Geometry: final body of the model. Coordinates: model frame, mm. Face numbers are marked on the shaded views. Give positions to 0.01 mm unless a question says otherwise; leave off trailing zeros. Order: outer loops, then holes, each group sorted by start corner. A loop starts at its lowest first (then second) coordinate and runs counter-clockwise, first axis right, second up. Notation, with made-up numbers: M 6.5,28 L 30.5,28 A29 cw 30.5,48 Z; hole C -3.5,34 d5. An arc over 180 degrees is marked long. Use CSV: the item, a comma, the result in double quotes.
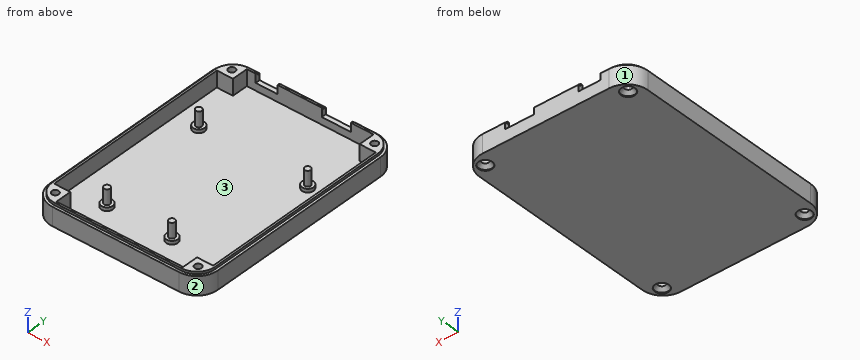
```python
from build123d import *

# Parameters (mm, degrees)
F1_DEPTH  = 2
F2_R      = 2.5
F3_DEPTH  = 1.5
F4_R      = 1.3
F5_DEPTH  = 1.5
F7_DEPTH  = 7
F8_R      = 1.5
F9_DEPTH  = 10
F10_W     = 12.6
F10_H     = 2
F10_W_2   = 9.5
F11_DEPTH = 3.8
F12_R     = 3
F13_DEPTH = 0.4
F14_SIZE  = 1.49999
F15_W     = 19.2
F15_H     = 1.1
F16_DEPTH = 1
F17_DEPTH = 5


# Not quite as in the source:
# - a fillet or chamfer is up to 0.001 mm smaller than in the source, because OpenCascade refuses the exact size


with BuildPart() as f1:
    # F0 (on Top) → F1 (new body)
    with BuildSketch(Plane.XY):
        with BuildLine():
            Line((27.5, 63.5), (-27.5, 63.5))
            ThreePointArc((-27.5, 63.5), (-33.8639610307, 60.8639610307), (-36.5, 54.5))
            Line((-36.5, 54.5), (-36.5, -27.5))
            ThreePointArc((-36.5, -27.5), (-33.8639610307, -33.8639610307), (-27.5, -36.5))
            Line((-27.5, -36.5), (27.5, -36.5))
            ThreePointArc((27.5, -36.5), (33.8639610307, -33.8639610307), (36.5, -27.5))
            Line((36.5, -27.5), (36.5, 54.5))
            ThreePointArc((36.5, 54.5), (33.8639610307, 60.8639610307), (27.5, 63.5))
        make_face()
    extrude(amount=F1_DEPTH)

    # F2 (on face) → F3 (join)
    with BuildSketch(Plane.XY.offset(2)):
        with Locations((-19.24, -18.6)):
            Circle(F2_R)
        with Locations((8.96, -18.6)):
            Circle(F2_R)
        with Locations((24.16, 32.2)):
            Circle(F2_R)
        with Locations((-24.24, 33.5)):
            Circle(F2_R)
    extrude(amount=F3_DEPTH)

    # F4 (on face) → F5 (join)
    with BuildSketch(Plane.XY.offset(3.5)):
        with Locations((-19.24, -18.6)):
            Circle(F4_R)
        with Locations((8.96, -18.6)):
            Circle(F4_R)
        with Locations((24.16, 32.2)):
            Circle(F4_R)
        with Locations((-24.24, 33.5)):
            Circle(F4_R)
    extrude(amount=F5_DEPTH)

    # F6 (on face) → F7 (join)
    with BuildSketch(Plane.XY.offset(2)):
        with BuildLine():
            Line((27.5, 63.5), (-27.5, 63.5))
            ThreePointArc((-27.5, 63.5), (-33.8639610307, 60.8639610307), (-36.5, 54.5))
            Line((-36.5, 54.5), (-36.5, -27.5))
            ThreePointArc((-36.5, -27.5), (-33.8639610307, -33.8639610307), (-27.5, -36.5))
            Line((-27.5, -36.5), (27.5, -36.5))
            ThreePointArc((27.5, -36.5), (33.8639610307, -33.8639610307), (36.5, -27.5))
            Line((36.5, -27.5), (36.5, 54.5))
            ThreePointArc((36.5, 54.5), (33.8639610307, 60.8639610307), (27.5, 63.5))
        make_face()
        Polygon((-27.5, 54.5), (-27.5, 61.5), (27.5, 61.5), (27.5, 54.5), (34.5, 54.5), (34.5, -27.5), (27.5, -27.5), (27.5, -34.5), (-27.5, -34.5), (-27.5, -27.5), (-34.5, -27.5), (-34.5, 54.5), align=None, mode=Mode.SUBTRACT)
    extrude(amount=F7_DEPTH)

    # F8 (on face) → F9 (cut)
    with BuildSketch(Plane.XY.offset(9)):
        with Locations((-31, 58)):
            Circle(F8_R)
        with Locations((31, 58)):
            Circle(F8_R)
        with Locations((-31, -31)):
            Circle(F8_R)
        with Locations((31, -31)):
            Circle(F8_R)
    extrude(amount=-F9_DEPTH, mode=Mode.SUBTRACT)

    # F10 (on face) → F11 (cut)
    with BuildSketch(Plane.XY.offset(9)):
        with Locations((11.36, 62.5)):
            Rectangle(F10_W, F10_H)
        with Locations((-18.89, 62.5)):
            Rectangle(F10_W_2, F10_H)
    extrude(amount=-F11_DEPTH, mode=Mode.SUBTRACT)

    # F12 (on face) → F13 (cut)
    with BuildSketch(Plane(origin=(0, 0, 0), x_dir=(1, 0, 0), z_dir=(0, 0, -1))):
        with Locations((31, -58)):
            Circle(F12_R)
        with Locations((-31, -58)):
            Circle(F12_R)
        with Locations((-31, 31)):
            Circle(F12_R)
        with Locations((31, 31)):
            Circle(F12_R)
    extrude(amount=-F13_DEPTH, mode=Mode.SUBTRACT)

    # F14 (size 1.5 in the source; OpenCascade refuses exactly that, so slightly less here)
    f14_edges = [f1.edges().sort_by_distance(p)[0] for p in [
        (29.5, 58, 0.4),
        (-32.5, 58, 0.4),
        (29.5, -31, 0.4),
        (-32.5, -31, 0.4),
    ]]
    chamfer(f14_edges, length=F14_SIZE)

    # F15 (on face) → F16 (cut)
    with BuildSketch(Plane.XY.offset(9)):
        with BuildLine():
            Line((-23.64, 63.5), (-27.5, 63.5))
            ThreePointArc((-27.5, 63.5), (-33.8639610307, 60.8639610307), (-36.5, 54.5))
            Line((-36.5, 54.5), (-36.5, -27.5))
            ThreePointArc((-36.5, -27.5), (-33.8639610307, -33.8639610307), (-27.5, -36.5))
            Line((-27.5, -36.5), (27.5, -36.5))
            ThreePointArc((27.5, -36.5), (33.8639610307, -33.8639610307), (36.5, -27.5))
            Line((36.5, -27.5), (36.5, 54.5))
            ThreePointArc((36.5, 54.5), (33.8639610307, 60.8639610307), (27.5, 63.5))
            Line((27.5, 63.5), (17.66, 63.5))
            Line((17.66, 63.5), (17.66, 62.4))
            Line((17.66, 62.4), (27.5, 62.4))
            ThreePointArc((27.5, 62.4), (33.0861435714, 60.0861435714), (35.4, 54.5))
            Line((35.4, 54.5), (35.4, -27.5))
            ThreePointArc((35.4, -27.5), (33.0861435714, -33.0861435714), (27.5, -35.4))
            Line((27.5, -35.4), (-27.5, -35.4))
            ThreePointArc((-27.5, -35.4), (-33.0861435714, -33.0861435714), (-35.4, -27.5))
            Line((-35.4, -27.5), (-35.4, 54.5))
            ThreePointArc((-35.4, 54.5), (-33.0861435714, 60.0861435714), (-27.5, 62.4))
            Line((-27.5, 62.4), (-23.64, 62.4))
            Line((-23.64, 62.4), (-23.64, 63.5))
        make_face()
        with Locations((-4.54, 62.95)):
            Rectangle(F15_W, F15_H)
    extrude(amount=-F16_DEPTH, mode=Mode.SUBTRACT)

    # F17 (add): faces of the model
    f17_faces = [f1.faces().sort_by_distance(p)[0] for p in [
        (-19.24, -18.6, 5),
        (8.96, -18.6, 5),
        (24.16, 32.2, 5),
        (-24.24, 33.5, 5),
    ]]
    extrude(f17_faces, amount=F17_DEPTH)


solid = f1.part
```
1. Pin query (flat end, axial travel): pin 1 Ø5.5 at (x, y) = (31, 58) entering from +Z; pin 2 Ø0.9 at (x, y) = (-7.5, 63) entering from +Z; pin 3 Ø1.6 at (y, z) = (63, 7) entering from +X. Return the tip coordinate at first contact, or that it passes through.
Answer:
pin 1,"z = 9"
pin 2,"z = 8"
pin 3,"x = 32.16"
2. Section D-D, the plane x = -8. Return the cut outline in (y, z).
Answer:
outline,"M -36.5,0 L 63.5,0 L 63.5,8 L 62.4,8 L 62.4,9 L 61.5,9 L 61.5,2 L -34.5,2 L -34.5,9 L -35.4,9 L -35.4,8 L -36.5,8 Z"
3. Section A-A, the plane x = 31. Give the number of separate pieces and of enclosed holes in the cut face, plus the area to 3 significant figures.
Answer:
separate pieces,"3"
enclosed holes,"0"
area,"250 mm2"
4. Section C-C, the plane y = -12. Return the cut outline in (x, z), plus the area to 3 significant figures.
Answer:
outline,"M -36.5,0 L 36.5,0 L 36.5,8 L 35.4,8 L 35.4,9 L 34.5,9 L 34.5,2 L -34.5,2 L -34.5,9 L -35.4,9 L -35.4,8 L -36.5,8 Z"
area,"172 mm2"
5. Line query: line 1 (Y direction, x = -3, z = 7.25); line 2 (Y direction, x = -31, z = 7.25); line 3 (X direction, y = 23.5, z = 3). Output: solid intervals per line, ascending.
Answer:
line 1,"-36.5 to -34.5, 61.5 to 63.5"
line 2,"-35.79 to -32.5, -29.5 to -27.5, 54.5 to 56.5, 59.5 to 62.79"
line 3,"-36.5 to -34.5, 34.5 to 36.5"
6. Pull-direction query (X, two-part tool) for the marked faces 1, 2 and 3; classes: +X half, -X half, draft (parallel to the pull), parting line (faces both ways), or undercut.
Answer:
face 1,"-X half"
face 2,"+X half"
face 3,"undercut"
